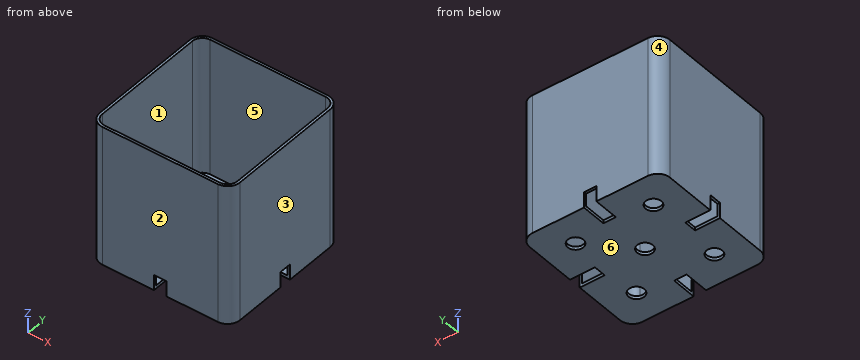
```python
from build123d import *

# Parameters (mm, degrees)
PAD_DEPTH       = 45
POCKET_DEPTH    = 44
SKETCH002_R     = 2.5
SKETCH002_W     = 4
SKETCH002_H     = 8
SKETCH002_W_2   = 8
SKETCH002_H_2   = 4
POCKET001_DEPTH = 5


with BuildPart() as part:
    # Sketch → Pad (new body)
    with BuildSketch(Plane.XY):
        with BuildLine():
            Line((4, 0), (41, 0))
            ThreePointArc((41, 0), (43.828427, 1.171573), (45, 4))
            Line((45, 4), (45, 41))
            ThreePointArc((45, 41), (43.828427, 43.828427), (41, 45))
            Line((41, 45), (4, 45))
            ThreePointArc((4, 45), (1.171573, 43.828427), (0, 41))
            Line((0, 41), (0, 4))
            ThreePointArc((0, 4), (1.171573, 1.171573), (4, 0))
        make_face()
    extrude(amount=PAD_DEPTH)

    # Sketch001 (on Face10 of Pad) → Pocket (cut)
    with BuildSketch(Plane.XY.offset(45)):
        with BuildLine():
            Line((4, 0.8), (41, 0.8))
            ThreePointArc((41, 0.8), (43.262742, 1.737258), (44.2, 4))
            Line((44.2, 4), (44.2, 41))
            ThreePointArc((44.2, 41), (43.262742, 43.262742), (41, 44.2))
            Line((41, 44.2), (4, 44.2))
            ThreePointArc((4, 44.2), (1.737258, 43.262742), (0.8, 41))
            Line((0.8, 41), (0.8, 4))
            ThreePointArc((0.8, 4), (1.737258, 1.737258), (4, 0.8))
        make_face()
    extrude(amount=-POCKET_DEPTH, mode=Mode.SUBTRACT)

    # Sketch002 (on Face4 of Pocket) → Pocket001 (cut)
    with BuildSketch(Plane(origin=(0, 0, 0), x_dir=(1, 0, 0), z_dir=(0, 0, -1))):
        with Locations((10, -10)):
            Circle(SKETCH002_R)
        with Locations((22.5, -22.5)):
            Circle(SKETCH002_R)
        with Locations((35, -10)):
            Circle(SKETCH002_R)
        with Locations((35, -35)):
            Circle(SKETCH002_R)
        with Locations((10, -35)):
            Circle(SKETCH002_R)
        with Locations((22.5, -4)):
            Rectangle(SKETCH002_W, SKETCH002_H)
        with Locations((4, -22.5)):
            Rectangle(SKETCH002_W_2, SKETCH002_H_2)
        with Locations((41, -22.5)):
            Rectangle(SKETCH002_W_2, SKETCH002_H_2)
        with Locations((22.5, -41)):
            Rectangle(SKETCH002_W, SKETCH002_H)
    extrude(amount=-POCKET001_DEPTH, mode=Mode.SUBTRACT)


solid = part.part
```
CAD build for the part. Positions are in the model's coordinates, mm. Face numbers are marked on the shaded views. A direction names the side the tool comes from. Round coordinates to 2 decimals unless told otherwise and drop trailing zeros. Order: outer loops, then holes, each group sorted by start corner. A loop starts at its lowest first (then second) coordinate and runs counter-clockwise, first axis right, second up.
Item 1: Mould opens along X. For the marked faces 1, 2, 3 and 4 say: pulls with the +X half, pulls with the -X half, needs draft (parallel to the pull), parting line crosses it, or undercut.
Item 2: Probe line 1 along Y through (x, z) = (10, 0.6); line 2 along Y through (x, z) = (41, 15.5). List the from-to ranges inside material, lowest first.
Item 3: Saw through at A-A on y = 22.5. Write the cut outline in (x, z), then the cut area to 3 significant figures.
Item 4: Saw through at C-C on x = 10. Write the cut outline in (y, z), then the cut area to 3 significant figures.
Item 5: Tool access for the marked faces 5 and 6: list every direction of +Z, -Z, +X, -X, +Y, -Y with a clear straight run to the whole face (end or side of a thin tool).
Item 6: Pin check, flat tips, straight feed: pin 1 (0.8 mm diameter, centred on y = 22.5, z = 0.5, fed in from -X); pin 2 (10 mm diameter, centred on x = 24.5, y = 17.5, fed in from +Z). Stop position of each tip, or through.
Item 7: Saw through at B-B on z = 24.5. Write the cut outline in (x, y), then the cut area to 3 significant figures.
Reported:
1. face 1: undercut
1. face 2: needs draft
1. face 3: pulls with the +X half
1. face 4: pulls with the -X half
2. line 1: y = 0 to 7.5, 12.5 to 32.5, 37.5 to 45
2. line 2: y = 0 to 0.8, 44.2 to 45
3. outline: (0, 5) - (0.8, 5) - (0.8, 45) - (0, 45) - close; (8, 0) - (20, 0) - (20, 1) - (8, 1) - close; (25, 0) - (37, 0) - (37, 1) - (25, 1) - close; (44.2, 5) - (45, 5) - (45, 45) - (44.2, 45) - close
3. area: 88.0 mm2
4. outline: (0, 0) - (7.5, 0) - (7.5, 1) - (0.8, 1) - (0.8, 45) - (0, 45) - close; (12.5, 0) - (32.5, 0) - (32.5, 1) - (12.5, 1) - close; (37.5, 0) - (45, 0) - (45, 45) - (44.2, 45) - (44.2, 1) - (37.5, 1) - close
4. area: 105 mm2
5. face 5: +Z
5. face 6: -Z, +X, -X, +Y, -Y
6. pin 1: stops at x = 8
6. pin 2: stops at z = 1
7. outline: (0, 4) arc R4 ccw to (4, 0) - (41, 0) arc R4 ccw to (45, 4) - (45, 41) arc R4 ccw to (41, 45) - (4, 45) arc R4 ccw to (0, 41) - close; hole (0.8, 4) arc R3.2 ccw to (4, 0.8) - (41, 0.8) arc R3.2 ccw to (44.2, 4) - (44.2, 41) arc R3.2 ccw to (41, 44.2) - (4, 44.2) arc R3.2 ccw to (0.8, 41) - close
7. area: 136 mm2
